```python
from build123d import *

# Parameters (mm, degrees)
F0_R      = 68.2625
F0_R_2    = 7.14375
F0_R_3    = 19.05
F1_DEPTH  = 31.75
F2_R      = 30.95625
F3_DEPTH  = 8.89
F4_R      = 44.45
F4_R_2    = 19.05
F5_DEPTH  = 88.9
F7_DEPTH  = 120.651
F8_SIZE   = 0.762
F9_R      = 1.5875
F10_DEPTH = 76.2


with BuildPart() as f1:
    # F0 (on Top) → F1 (new body)
    with BuildSketch(Plane.XY):
        Circle(F0_R)
        with Locations((-28.575, -49.493352)):
            Circle(F0_R_2, mode=Mode.SUBTRACT)
        with Locations((28.575, -49.493352)):
            Circle(F0_R_2, mode=Mode.SUBTRACT)
        with Locations((-57.15, 0)):
            Circle(F0_R_2, mode=Mode.SUBTRACT)
        with Locations((-28.575, 49.493352)):
            Circle(F0_R_2, mode=Mode.SUBTRACT)
        Circle(F0_R_3, mode=Mode.SUBTRACT)
        with Locations((57.15, 0)):
            Circle(F0_R_2, mode=Mode.SUBTRACT)
        with Locations((28.575, 49.493352)):
            Circle(F0_R_2, mode=Mode.SUBTRACT)
    extrude(amount=F1_DEPTH)

    # F2 (on face) → F3 (cut)
    with BuildSketch(Plane.XY.offset(31.75)):
        Circle(F2_R)
    extrude(amount=-F3_DEPTH, mode=Mode.SUBTRACT)

    # F4 (on face) → F5 (join)
    with BuildSketch(Plane(origin=(0, 0, 0), x_dir=(1, 0, 0), z_dir=(0, 0, -1))):
        Circle(F4_R)
        Circle(F4_R_2, mode=Mode.SUBTRACT)
    extrude(amount=F5_DEPTH)

    # F6 (on face) → F7 (cut, through all)
    with BuildSketch(Plane(origin=(0, 0, -88.9), x_dir=(1, 0, 0), z_dir=(0, 0, -1))):
        Polygon((4.7625, -10.517543), (0, -10.517543), (0, -19.05), (0, -23.8125), (4.7625, -23.8125), align=None)
        Polygon((0, -19.05), (0, -10.517543), (-4.7625, -10.517543), (-4.7625, -23.8125), (0, -23.8125), align=None)
    extrude(amount=-F7_DEPTH, mode=Mode.SUBTRACT)

    # F8
    f8_edges = [f1.edges().sort_by_distance(p)[0] for p in [
        (-68.2625, 0, 31.75),
        (-68.2625, 0, 0),
        (-30.95625, 0, 31.75),
        (-44.45, 0, -88.9),
    ]]
    chamfer(f8_edges, length=F8_SIZE)

    # F9 (on Front) → F10 (cut)
    with BuildSketch(Plane.XZ):
        with Locations((0, -69.271334)):
            Circle(F9_R)
    extrude(amount=-F10_DEPTH, mode=Mode.SUBTRACT)


solid = f1.part
```
Design review of the part built by this model. Coordinates are the model's own, in mm. A direction names the side the tool comes from. Give positions to 0.01 mm unless a question says otherwise; leave off trailing zeros. Loops run counter-clockwise (first coordinate to the right, second up) from the corner with the lowest first, then second, coordinate; pieces in that order, holes last. Notation, with made-up numbers: (56, 78.5) -> (107, 78.5) arc R23 ccw to (107, 108.5) -> close; hole circle Ø6 at (46.25, 71). An arc over 180 degrees is marked (long way). Write each question's results on one line, items separated by ' | '.
Q1. Take a section at A-A, the plane y = 0. Give the number of separate pieces and of enclosed holes in the cut face, plus the area to 3 significant figures.
Reply:
separate pieces: 4 | enclosed holes: 0 | area: 6,520 mm²
Q2. The part is to be moulded in two halves that separate along X. For faces 4 (the face through (4.762, 21, -34)), 5 (the face through (19, 9, -88.9)), 6 (the face through (0, 23.812, -34)), 7 (the face through (42.397, -13.352, -43.452)), say which applies: +X half, -X half, draft (parallel to the pull), parting line (faces both ways), or undercut.
Reply:
face 4: undercut | face 5: draft | face 6: undercut | face 7: parting line
Q3. Take a section at B-B, the plane z = -53. Write out the cut boundary in (x, y).
Reply:
outline: circle Ø88.9 at (0, 0); hole (-4.76, 18.45) arc R19.05 ccw (long way) to (4.76, 18.45) -> (4.76, 23.81) -> (-4.76, 23.81) -> close
Q4. Machinability: for faces 1 (the face through (-68.196, 3.001, 15.663)), 2 (the face through (-6.71, -30.22, 26.98)), 3 (the face through (44, -14, 0)), which of the approach directions +Z, -Z, +X, -X, +Y, -Y give a long, thin tool a straight path to every point of the face, cutting with its end or side? Answer none if there is none.
Reply:
face 1: +Z, -Z | face 2: +Z | face 3: -Z
Q5. For pin 1 Ø8.5 at (x, y) = (-57.15, 0) entering from +Z; pin 2 Ø6 at (x, y) = (-45.5, 34) entering from -Z; pin 3 Ø5 at (x, z) = (0.5, -19) entering from -Y; pin 4 Ø3 at (x, z) = (0, -69.27) entering from +Y, all flat-tipped, find the tip position at first contact; note any pin that passes through.
Reply:
pin 1: passes through | pin 2: stops at z = 0 | pin 3: stops at y = -44.45 | pin 4: stops at y = -18.99
Q6. Wall thickness on L1, parallel to X at y = 53.5, z = 9; L2, parallel to Z at x = -18, y = -14.5; L3, parallel to Y at x = 57.15, z = 8: over which ranges is each line inside the solid? List them lowest first.
Reply:
L1: x = -42.4 to -34.49, -22.66 to 22.66, 34.49 to 42.4 | L2: z = -88.9 to 22.86 | L3: y = -37.33 to -7.14, 7.14 to 37.33
